Geometry: final body of the model. Coordinates: model frame, mm. Face numbers are marked on the shaded views. A direction names the side the tool comes from. Round coordinates to 2 decimals unless told otherwise and drop trailing zeros. Loops run counter-clockwise (first coordinate to the right, second up) from the corner with the lowest first, then second, coordinate; pieces in that order, holes last. Notation, with made-up numbers: (68, 13.5) -> (102, 13.5) arc R32 cw to (102, 43.5) -> close; hole circle Ø9 at (41.5, 63). An arc over 180 degrees is marked (long way). Answer in a Markdown table with one row per item.
Solid Edge part; units mm, degrees
sketch "Sketch1" plane through (0, 0, 0) normal (0, -1, 0) x (1, 0, 0)
  circle A0 centre (12.343, 25.5757) radius 1.65
  arc A1 (2.343, 63.5757) -> (22.343, 63.5757) centre (12.343, 63.5757) cw
  line L0 (22.343, 63.5757) -> (22.343, 25.5757)
  arc A2 (22.343, 25.5757) -> (2.343, 25.5757) centre (12.343, 25.5757) cw
  line L1 (2.343, 25.5757) -> (2.343, 63.5757)
  circle A3 centre (12.343, 63.5757) radius 1.65
extrude "Protrusion1" add sketch "Sketch1" against normal blind 12
sketch "Sketch2" plane through (12.343, 6, 73.5757) normal (0, 0, 1) x (0, -1, 0)
  line L0 (2.2, -10.2) -> (2.2, 10.2)
  line L1 (2.2, 10.2) -> (-2.2, 10.2)
  line L2 (-2.2, 10.2) -> (-2.2, -10.2)
  line L3 (-2.2, -10.2) -> (2.2, -10.2)
extrude "ExtrudedCutout_1" cut sketch "Sketch2" against normal blind 20
sketch "Sketch3" plane through (12.343, 6, 15.5757) normal (0, 0, -1) x (0, -1, 0)
  line L0 (2.2, 10.2) -> (-2.2, 10.2)
  line L1 (-2.2, 10.2) -> (-2.2, -10.2)
  line L2 (-2.2, -10.2) -> (2.2, -10.2)
  line L3 (2.2, -10.2) -> (2.2, 10.2)
extrude "ExtrudedCutout_7" cut sketch "Sketch3" against normal blind 20
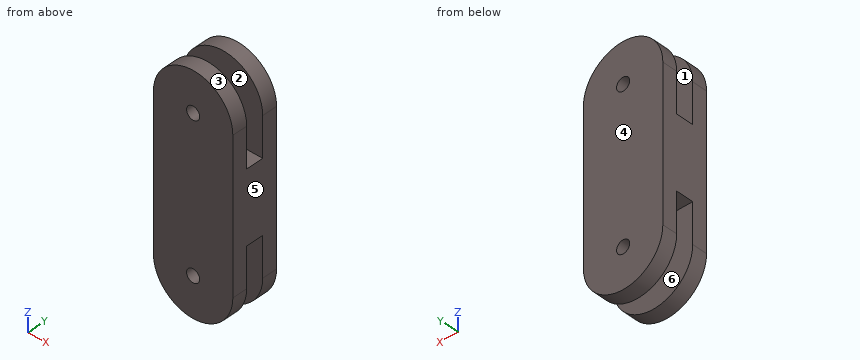
Item 1: Cut plane B-B (x = 12.75). Output: boundary loops of the cut face in (y, z).
Answer:
| item | result |
|---|---|
| outline | (0, 15.58) -> (3.8, 15.58) -> (3.8, 23.98) -> (0, 23.98) -> close; (0, 27.17) -> (3.8, 27.17) -> (3.8, 35.58) -> (8.2, 35.58) -> (8.2, 27.17) -> (12, 27.17) -> (12, 61.98) -> (8.2, 61.98) -> (8.2, 53.58) -> (3.8, 53.58) -> (3.8, 61.98) -> (0, 61.98) -> close; (0, 65.17) -> (3.8, 65.17) -> (3.8, 73.57) -> (0, 73.57) -> close; (8.2, 15.58) -> (12, 15.58) -> (12, 23.98) -> (8.2, 23.98) -> close; (8.2, 65.17) -> (12, 65.17) -> (12, 73.57) -> (8.2, 73.57) -> close |
Item 2: Line query: probe 1 along Y at (x, z) = (20.25, 34.5); probe 2 along Z at (x, y) = (13.5, 11); probe 3 along Z at (x, y) = (11.75, 9). Output: solid intervals per line, ascending. Write a range as [from, to].
Answer:
| item | result |
|---|---|
| probe 1 | y = [0, 3.8], [8.2, 12] |
| probe 2 | z = [15.64, 24.4], [26.75, 62.4], [64.75, 73.51] |
| probe 3 | z = [15.59, 24.04], [27.12, 62.04], [65.12, 73.56] |
Item 3: Pin query (flat end, axial travel): pin 1 Ø3.5 at (x, y) = (14, 7) entering from -Z; pin 2 Ø5.5 at (x, z) = (12.34, 25.58) entering from -Y; pin 3 Ø2.5 at (x, z) = (12.34, 25.58) entering from -Y; pin 4 Ø1.3 at (x, y) = (9.5, 7) entering from +Z. Return the tip coordinate at first contact, or that it passes through.
Answer:
| item | result |
|---|---|
| pin 1 | stops at z = 15.58 |
| pin 2 | stops at y = 0 |
| pin 3 | passes through |
| pin 4 | stops at z = 53.58 |
Item 4: Cut plane A-A (z = 54.5). Output: boundary loops of the cut face in (x, y), then the cut area to 3 significant figures.
Answer:
| item | result |
|---|---|
| outline | (2.34, 0) -> (22.34, 0) -> (22.34, 3.8) -> (2.34, 3.8) -> close; (2.34, 8.2) -> (22.34, 8.2) -> (22.34, 12) -> (2.34, 12) -> close |
| area | 152 mm² |
Item 5: Draft query along Y for the marked faces 1, 2, 3 and 4. Return one class per face: pulls with the +Y half, pulls with the -Y half, needs draft (parallel to the pull), parting line crosses it, or undercut.
Answer:
| item | result |
|---|---|
| face 1 | undercut |
| face 2 | undercut |
| face 3 | needs draft |
| face 4 | pulls with the +Y half |
Item 6: Reachability of the marked faces 5 and 6 from +Z, -Z, +X, -X, +Y, -Y: full face, straight path, thin tool, end or side. Return the list, or none.
Answer:
| item | result |
|---|---|
| face 5 | +Z, -Z, +X, +Y, -Y |
| face 6 | -Z, +X, -X |
Item 7: Cut plane C-C (y = 9.25). Output: boundary loops of the cut face in (x, z).
Answer:
| item | result |
|---|---|
| outline | (2.34, 25.58) arc R10 ccw to (22.34, 25.58) -> (22.34, 63.58) arc R10 ccw to (2.34, 63.58) -> close; hole circle Ø3.3 at (12.34, 25.58); hole circle Ø3.3 at (12.34, 63.58) |
Item 8: Cut plane D-D (z = 70). Output: boundary loops of the cut face in (x, y).
Answer:
| item | result |
|---|---|
| outline | (4.68, 0) -> (20.01, 0) -> (20.01, 3.8) -> (4.68, 3.8) -> close; (4.68, 8.2) -> (20.01, 8.2) -> (20.01, 12) -> (4.68, 12) -> close |
